```python
from build123d import *

# Parameters (mm, degrees)
SKETCH2_R           = 2.15
BOSS_EXTRUDE1_DEPTH = 78.1
CUT_EXTRUDE1_DEPTH  = 21
CUT_EXTRUDE2_DEPTH  = 21


with BuildPart() as part:
    # Sketch2 → Boss-Extrude1 (new body, symmetric)
    with BuildSketch(Plane.XY):
        Polygon((-2.5, 10), (-2.5, 8.2), (-6.927207794, 8.2), (-2.677207794, 3.95), (2.677207794, 3.95), (6.927207794, 8.2), (2.5, 8.2), (2.5, 10), (10, 10), (10, 2.5), (8.2, 2.5), (8.2, 6.927207794), (3.95, 2.677207794), (3.95, -2.677207794), (8.2, -6.927207794), (8.2, -2.5), (10, -2.5), (10, -10), (2.5, -10), (2.5, -8.2), (6.927207794, -8.2), (2.677207794, -3.95), (-2.677207794, -3.95), (-6.927207794, -8.2), (-2.5, -8.2), (-2.5, -10), (-10, -10), (-10, -2.5), (-8.2, -2.5), (-8.2, -6.927207794), (-3.95, -2.677207794), (-3.95, 2.677207794), (-8.2, 6.927207794), (-8.2, 2.5), (-10, 2.5), (-10, 10), align=None)
        Circle(SKETCH2_R, mode=Mode.SUBTRACT)
    extrude(amount=BOSS_EXTRUDE1_DEPTH, both=True)

    # Sketch3 → Cut-Extrude1 (cut, through all)
    with BuildSketch(Plane(origin=(0, 10, 0), x_dir=(1, 0, 0), z_dir=(0, 1, 0))):
        Polygon((-10, -78.1), (10, -78.1), (-10, -68.773846837), align=None)
    extrude(amount=-CUT_EXTRUDE1_DEPTH, mode=Mode.SUBTRACT)

    # Sketch4 → Cut-Extrude2 (cut, through all)
    with BuildSketch(Plane(origin=(0, 10, 0), x_dir=(1, 0, 0), z_dir=(0, 1, 0))):
        Polygon((10, 78.1), (-10, 78.1), (-10, 70.820595315), align=None)
    extrude(amount=-CUT_EXTRUDE2_DEPTH, mode=Mode.SUBTRACT)


solid = part.part
```
For this review, take the finished solid that the model builds, in its own axes (mm). Round coordinates to 2 decimals unless told otherwise and drop trailing zeros. Write each loop counter-clockwise with the first axis right and the second up, starting at its lowest first coordinate (ties: lowest second). Pieces come first, ordered by that corner, then holes.
1) Take a section at B-B on x = 0. Give the boundary of the cut face in (y, z).
Answer below:
outline: (-3.95, -74.46) - (-2.15, -74.46) - (-2.15, 73.44) - (-3.95, 73.44) - close; (2.15, -74.46) - (3.95, -74.46) - (3.95, 73.44) - (2.15, 73.44) - close
2) Mouldability with a two-part tool opening along Y and no side actions: class faces 1 (the face through (-4.83, 6.1, 0.37)), 2 (the face through (0.14, 2.36, 73.5)), 3 (the face through (6, -10, 1)) as +Y half, -Y half, draft (parallel to the pull), parting line (faces both ways), or undercut.
Answer below:
face 1: undercut
face 2: draft
face 3: -Y half
3) Take a section at A-A on y = 0. Give the boundary of the cut face in (x, z) (3 decimals), then the cut area to 3 significant figures.
Answer below:
outline: (-3.95, -73.023) - (-2.15, -73.678) - (-2.15, 72.434) - (-3.95, 71.595) - close; (2.15, -75.243) - (3.95, -75.898) - (3.95, 75.279) - (2.15, 74.439) - close
area: 532 mm2
4) Insertion check: pin 1 Ø1 at (x, z) = (1.5, -1.5) entering from -Y; pin 2 Ø5 at (x, y) = (0, 0) entering from -Z; pin 3 Ø1 at (x, z) = (1, -9) entering from +Y. Each pin has a flat end and moves straight along its axis. Give the tip position at first contact, or say it passes through.
Answer below:
pin 1: stops at y = -3.95
pin 2: stops at z = -75.37
pin 3: stops at y = 3.95
5) For line 1 along X through (y, z) = (0, 26.5); line 2 along X through (y, z) = (6.25, -40.5), list the stretches that pass through material, from the lowest coordinate up.
Answer below:
line 1: x = -3.95 to -2.15, 2.15 to 3.95
line 2: x = -10 to -8.2, -7.52 to -4.98, 4.98 to 7.52, 8.2 to 10
